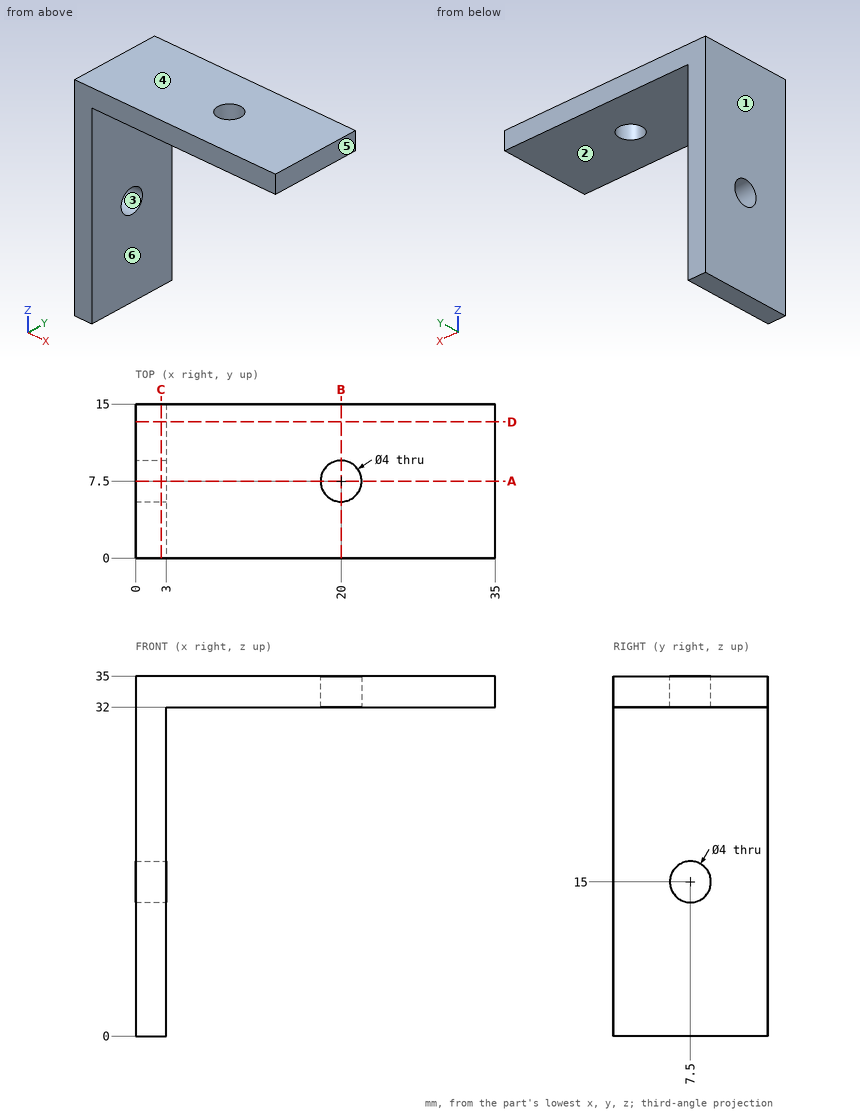
Input: dimensioned drawing with shaded views. Units: mm. Origin: part minimum x, y, z. A direction names the side the tool comes from. Coordinates: 2 decimals unless noted, no trailing zeros. Write each loop counter-clockwise with the first axis right and the second up, starting at its lowest first coordinate (ties: lowest second). Pieces come first, ordered by that corner, then holes. Notation, with made-up numbers: M 41,-2.75 L 99,-2.75 A9 ccw 99,3.25 Z; hole C 67,31.25 d7. An arc over 180 degrees is marked long. Use one line per item in the form item = value.
Q1. Section B-B (x = 20). Return loops of the section in (y, z).
Answer below:
outline = M 0,32 L 5.5,32 L 5.5,35 L 0,35 Z; M 9.5,32 L 15,32 L 15,35 L 9.5,35 Z
Q2. Set-up query: the marked faces 5 and 6. Return all of +Z, -Z, +X, -X, +Y, -Y with unobstructed straight access to the full face (end or side cutting, diameter ignored); none if empty.
Answer below:
face_5 = +Z, -Z, +X, +Y, -Y
face_6 = -Z, +X, +Y, -Y
Q3. First-contact query: pin 1 (8 mm diameter, centred on x = 7.5, z = 19, fed in from -Y) (3 decimals); pin 2 (7.5 mm diameter, centred on y = 10, z = 8, fed in from +X); pin 3 (4.5 mm diameter, centred on x = 22.5, y = 6.5, fed in from -Z). Flat tips, straight axial feed; report the tip coordinate or a pass-through.
Answer below:
pin_1 = through
pin_2 = 3
pin_3 = 32
Q4. Material intervals for probe 1 along Y at (x, z) = (20, 33.95); probe 2 along Z at (x, y) = (4.5, 4.5); probe 3 along X at (y, z) = (11.5, 4), sorted ascending. Write a range as from..to.
Answer below:
probe_1 = 0..5.5, 9.5..15
probe_2 = 32..35
probe_3 = 0..3
Q5. Draft query along Z for the marked faces 1, 2, 3 and 4. Return one class per face: released by +Z, released by -Z, zero draft, split by the parting line, or undercut.
Answer below:
face_1 = zero draft
face_2 = released by -Z
face_3 = undercut
face_4 = released by +Z
Q6. Section A-A (y = 7.5). Return loops of the section in (x, z).
Answer below:
outline = M 0,0 L 3,0 L 3,13 L 0,13 Z; M 0,17 L 3,17 L 3,32 L 18,32 L 18,35 L 0,35 Z; M 22,32 L 35,32 L 35,35 L 22,35 Z
Q7. Section D-D (y = 13.25). Return loops of the section in (x, z), plus the area to 3 significant figures.
Answer below:
outline = M 0,0 L 3,0 L 3,32 L 35,32 L 35,35 L 0,35 Z
area = 201 mm²
Q8. Section C-C (x = 2.5). Return loops of the section in (y, z).
Answer below:
outline = M 0,0 L 15,0 L 15,35 L 0,35 Z; hole C 7.5,15 d4
